from build123d import *

# Parameters (mm, degrees)
SKETCH1_R           = 4
BOSS_EXTRUDE1_DEPTH = 6


with BuildPart() as part:
    # Sketch1 → Boss-Extrude1 (new body)
    with BuildSketch(Plane.XY):
        with BuildLine():
            Line((-200.213397345, 335.278845102), (-182.330447011, 344.688065085))
            ThreePointArc((-182.330447011, 344.688065085), (-177.281730902, 345.830599505), (-172.338147286, 344.295705283))
            Line((-172.338147286, 344.295705283), (-155.248048584, 333.513225991))
            ThreePointArc((-155.248048584, 333.513225991), (-151.734226698, 329.712176794), (-150.591692278, 324.663460686))
            Line((-150.591692278, 324.663460686), (-153.067482632, 261.612049424))
            Line((-153.067482632, 261.612049424), (-208.025131117, 263.770028338))
            Line((-208.025131117, 263.770028338), (-205.549340763, 326.8214396))
            ThreePointArc((-205.549340763, 326.8214396), (-204.014446541, 331.765023216), (-200.213397345, 335.278845102))
        make_face()
        with Locations((-178.467049866, 315.643862037)):
            Circle(SKETCH1_R, mode=Mode.SUBTRACT)
    extrude(amount=BOSS_EXTRUDE1_DEPTH)


solid = part.part
Verification items for the finished model (mm, model axes). Give positions to 0.01 mm unless a question says otherwise; leave off trailing zeros. Order: outer loops, then holes, each group sorted by start corner. A loop starts at its lowest first (then second) coordinate and runs counter-clockwise, first axis right, second up. Notation, with made-up numbers: (88, -3.5) -> (118, -3.5) arc R33 cw to (118, 25.5) -> close; hole circle Ø10 at (29.5, 21.5). An arc over 180 degrees is marked (long way). Answer as CSV lines item,"result".
Q1. Scan lines: probe 1 along Y at (x, z) = (-180.5, 4.8); probe 2 along X at (y, z) = (341, 2.25); probe 3 along X at (y, z) = (270, 4.85). Record each from-to range of solid material in increasing order.
Solutions:
probe 1,"y = 262.69 to 312.2, 319.09 to 345.43"
probe 2,"x = -189.34 to -167.11"
probe 3,"x = -207.78 to -152.74"
Q2. Depth check by flat-ended pin: pin 1 (3 mm diameter, centred on x = -201, z = 1.5, fed in from +Y); pin 2 (2 mm diameter, centred on y = 287.5, z = 3.5, fed in from +X); pin 3 (1 mm diameter, centred on y = 314.5, z = 3.5, fed in from +X); pin 4 (5 mm diameter, centred on x = -178.47, y = 315.64, fed in from -Z). Enter the tip coordinate at first touch or a pass-through.
Solutions:
pin 1,"stops at y = 335.65"
pin 2,"stops at x = -152.01"
pin 3,"stops at x = -150.97"
pin 4,"passes through"
Q3. Sectioned sample at A-A on y = 314.5. Record the cut outline in (x, z).
Solutions:
outline,"(-206.03, 0) -> (-182.3, 0) -> (-182.3, 6) -> (-206.03, 6) -> close; (-174.63, 0) -> (-150.99, 0) -> (-150.99, 6) -> (-174.63, 6) -> close"
Q4. Sectioned sample at D-D on y = 331.5. Record the cut outline in (x, z), plus the area to 3 significant figures.
Solutions:
outline,"(-204.18, 0) -> (-152.94, 0) -> (-152.94, 6) -> (-204.18, 6) -> close"
area,"307 mm²"
Q5. Sectioned sample at B-B on z = 1.3. Record the cut outline in (x, y), plus the area to 3 significant figures.
Solutions:
outline,"(-208.03, 263.77) -> (-153.07, 261.61) -> (-150.59, 324.66) arc R10 ccw to (-155.25, 333.51) -> (-172.34, 344.3) arc R10 ccw to (-182.33, 344.69) -> (-200.21, 335.28) arc R10 ccw to (-205.55, 326.82) -> close; hole circle Ø8 at (-178.47, 315.64)"
area,"4,160 mm²"
Q6. Release check for a two-part mould opening along Y. For faces 1 (the flat face through (-163.91, 338.98, 2.96)), 2 (the flat face through (-179, 304, 6)), 3 (the cylindrical face through (-176.32, 319.02, 2.96)), 4 (the flat face through (-151.812, 293.579, 2.958)) record: +Y half, -Y half, draft (parallel to the pull), parting line (faces both ways), or undercut.
Solutions:
face 1,"+Y half"
face 2,"draft"
face 3,"undercut"
face 4,"-Y half"
Q7. Sectioned sample at C-C on x = -197.5. Record the cut outline in (y, z), plus the area to 3 significant figures.
Solutions:
outline,"(263.36, 0) -> (336.71, 0) -> (336.71, 6) -> (263.36, 6) -> close"
area,"440 mm²"
